```python
from build123d import *

# Parameters (mm, degrees)
ESQUISSE1_W             = 33
ESQUISSE1_H             = 33
BOSS_EXTRU_1_DEPTH      = 12.5
ESQUISSE3_R             = 2
ESQUISSE3_W             = 2.1
ESQUISSE3_H             = 2.8
ENL_V_MAT_EXTRU_1_DEPTH = 13.5
ESQUISSE2_R             = 1.2
ENL_V_MAT_EXTRU_3_DEPTH = 13.5
ESQUISSE5_W             = 20.32
ESQUISSE5_H             = 20.32
ENL_V_MAT_EXTRU_5_DEPTH = 10.5
ESQUISSE8_R             = 8
BOSS_EXTRU_4_DEPTH      = 12.5
D_GAGEMENT_M31_D        = 3.4
CHANFREIN1_SIZE         = 1
CHANFREIN2_SIZE         = 0.5


with BuildPart() as part:
    # Esquisse1 → Boss.-Extru.1 (new body)
    with BuildSketch(Plane.XY):
        Rectangle(ESQUISSE1_W, ESQUISSE1_H)
    extrude(amount=BOSS_EXTRU_1_DEPTH)

    # Esquisse3 → Enlèv. mat.-Extru.1 (cut, through all)
    with BuildSketch(Plane.XY.offset(12.5)):
        with Locations((0.25, 0)):
            Circle(ESQUISSE3_R)
        with Locations((-2.97, 0)):
            Rectangle(ESQUISSE3_W, ESQUISSE3_H)
    extrude(amount=-ENL_V_MAT_EXTRU_1_DEPTH, mode=Mode.SUBTRACT)

    # Esquisse2 → Enlèv. mat.-Extru.3 (cut, through all)
    with BuildSketch(Plane.XY.offset(12.5)):
        with BuildLine():
            Line((7.62, 8.82), (-7.62, 8.82))
            ThreePointArc((-7.62, 8.82), (-8.82, 7.62), (-7.62, 6.42))
            Line((-7.62, 6.42), (7.62, 6.42))
            ThreePointArc((7.62, 6.42), (8.82, 7.62), (7.62, 8.82))
        make_face()
        with Locations((7.62, -7.62)):
            Circle(ESQUISSE2_R)
        with Locations((-7.62, -7.62)):
            Circle(ESQUISSE2_R)
    extrude(amount=-ENL_V_MAT_EXTRU_3_DEPTH, mode=Mode.SUBTRACT)

    # Esquisse5 → Enlèv. mat.-Extru.5 (cut)
    with BuildSketch(Plane.XY.offset(12.5)):
        Rectangle(ESQUISSE5_W, ESQUISSE5_H)
    extrude(amount=-ENL_V_MAT_EXTRU_5_DEPTH, mode=Mode.SUBTRACT)

    # Esquisse8 → Boss.-Extru.4 (add)
    with BuildSketch(Plane(origin=(0, 0, 0), x_dir=(-1, 0, 0), z_dir=(0, 0, -1))):
        with BuildLine():
            Line((-10.491194523, 35.577324893), (-30.491194523, 35.577324893))
            ThreePointArc((-30.491194523, 35.577324893), (-27.133349226, 16.503433006), (-16.5, 0.31639001))
            Line((-16.5, 0.31639001), (-16.5, 16.5))
            Line((-16.5, 16.5), (-4.221778996, 16.5))
            ThreePointArc((-4.221778996, 16.5), (-9.129954495, 25.455844561), (-10.491194523, 35.577324893))
        make_face()
        with Locations((-20.024037982, 25.814414184)):
            Circle(ESQUISSE8_R, mode=Mode.SUBTRACT)
        with BuildLine():
            Line((44.278689278, 26.536687189), (63.501960696, 21.070416717))
            ThreePointArc((63.501960696, 21.070416717), (45.926381173, -4.33394458), (16.5, -13.734511563))
            Line((16.5, -13.734511563), (16.5, 6.257008408))
            ThreePointArc((16.5, 6.257008408), (33.880318455, 11.614983254), (44.278689278, 26.536687189))
        make_face()
    extrude(amount=-BOSS_EXTRU_4_DEPTH)

    # Dégagement M31 (through all)
    with Locations(Plane(origin=(-13.5, 13.5, 12.5), x_dir=(1, 0, 0), z_dir=(0, 0, 1))):
        with Locations((0, 0), (27, 0), (27, -27), (0, -27)):
            Hole(D_GAGEMENT_M31_D / 2)

    # Chanfrein1
    chanfrein1_edges = [part.edges().sort_by_distance(p)[0] for p in [
        (-11.8, -13.5, 0),
        (15.2, -13.5, 0),
        (15.2, 13.5, 0),
        (-11.8, 13.5, 0),
    ]]
    chamfer(chanfrein1_edges, length=CHANFREIN1_SIZE)

    # Chanfrein2
    chanfrein2_edges = [part.edges().sort_by_distance(p)[0] for p in [
        (6.42, -7.62, 0),
        (-8.82, -7.62, 0),
    ]]
    chamfer(chanfrein2_edges, length=CHANFREIN2_SIZE)


solid = part.part
```
Geometry: final body of the model. Coordinates: model frame, mm. A direction names the side the tool comes from. Coordinates: 2 decimals unless noted, no trailing zeros. Order: outer loops, then holes, each group sorted by start corner. A loop starts at its lowest first (then second) coordinate and runs counter-clockwise, first axis right, second up. Notation, with made-up numbers: (32, 24) - (40, 24) arc R20 cw to (40, 58) - close; hole circle Ø8 at (0.5, 72.25). An arc over 180 degrees is marked (long way). Return JSON: item names as keys, results as strings. Group by question number.
1. Pin query (flat end, axial travel): pin 1 (1 mm diameter, centred on x = -6, y = -4, fed in from +Z); pin 2 (1 mm diameter, centred on x = -3, z = 0.5, fed in from +Y); pin 3 (12 mm diameter, centred on x = -10, y = 1, fed in from +Z); pin 4 (2 mm diameter, centred on y = -0.5, z = 1, fed in from -X). Return the tip coordinate at first contact, or that it passes through.
2. Material intervals for line 1 along Y through (x, z) = (-7.62, 1.5); line 2 along Y through (x, z) = (0.25, 1.05); line 3 along Y through (x, z) = (1, 3.25), sorted ascending. Write a range as [from, to].
3. Cut plane A-A (x = 0.25). Output: boundary loops of the cut face in (y, z), plus the area to 3 significant figures.
4. Pull-direction query (Y, two-part tool) for faces 1 (the face through (-33.67, 11.463, 6.162)), 2 (the face through (-16.5, -15, 6)), 3 (the face through (0, -10.16, 7)); classes: pulls with the +Y half, pulls with the -Y half, needs draft (parallel to the pull), parting line crosses it, or undercut.
5. Set-up query: faces 4 (the face through (16.5, -8, 6)), 5 (the face through (0, -16.5, 6)), 6 (the face through (-3, -1.4, 1)), 7 (the face through (0, 10.16, 7)), 8 (the face through (-16.5, 11, 6)). Return all of +Z, -Z, +X, -X, +Y, -Y with unobstructed straight access to the full face (end or side cutting, diameter ignored); none if empty.
6. Cut plane D-D (y = 13.5). Output: boundary loops of the cut face in (x, z), plus the area to 3 significant figures.
7. Cut plane C-C (x = 13.5). Output: boundary loops of the cut face in (y, z), plus the area to 3 significant figures.
8. Cut plane B-B (y = 31). Output: boundary loops of the cut face in (x, z).
Resolved:
{
 "1": {"pin 1": "stops at z = 2", "pin 2": "stops at y = 16.5", "pin 3": "stops at z = 12.5", "pin 4": "stops at x = -51.5"},
 "2": {"line 1": "y = [-16.5, -8.82], [-6.42, 6.42], [8.82, 16.5]", "line 2": "y = [-16.5, -2], [2, 6.42], [8.82, 16.5]", "line 3": "y = [-16.5, -10.16], [10.16, 16.5]"},
 "3": {"outline": "(-16.5, 0) - (-2, 0) - (-2, 2) - (-10.16, 2) - (-10.16, 12.5) - (-16.5, 12.5) - close; (2, 0) - (6.42, 0) - (6.42, 2) - (2, 2) - close; (8.82, 0) - (16.5, 0) - (16.5, 12.5) - (10.16, 12.5) - (10.16, 2) - (8.82, 2) - close", "area": "186 mm²"},
 "4": {"face 1": "pulls with the +Y half", "face 2": "needs draft", "face 3": "undercut"},
 "5": {"face 4": "+Z, -Z, +X, -Y", "face 5": "+Z, -Z, +X, -X, -Y", "face 6": "+Z, -Z", "face 7": "+Z", "face 8": "+Z, -Z, +Y"},
 "6": {"outline": "(-60.64, 0) - (-36.19, 0) - (-36.19, 12.5) - (-60.64, 12.5) - close; (-16.5, 0) - (-16.2, 0) - (-15.2, 1) - (-15.2, 12.5) - (-16.5, 12.5) - close; (-11.8, 1) - (-10.8, 0) - (10.8, 0) - (11.8, 1) - (11.8, 12.5) - (-11.8, 12.5) - close; (15.2, 1) - (16.2, 0) - (25.82, 0) - (25.82, 12.5) - (15.2, 12.5) - close", "area": "748 mm²"},
 "7": {"outline": "(-16.5, 0) - (-16.2, 0) - (-15.2, 1) - (-15.2, 12.5) - (-16.5, 12.5) - close; (-11.8, 1) - (-10.8, 0) - (10.8, 0) - (11.8, 1) - (11.8, 12.5) - (-11.8, 12.5) - close; (15.2, 1) - (16.2, 0) - (21.18, 0) - (21.18, 12.5) - (15.2, 12.5) - close; (30.44, 0) - (35.58, 0) - (35.58, 12.5) - (30.44, 12.5) - close", "area": "448 mm²"},
 "8": {"outline": "(10.35, 0) - (13.93, 0) - (13.93, 12.5) - (10.35, 12.5) - close; (26.12, 0) - (30.41, 0) - (30.41, 12.5) - (26.12, 12.5) - close"}
}
